from build123d import *
from OCP.BRepFilletAPI import BRepFilletAPI_MakeChamfer

# Parameters (mm, degrees)
BOSS_EXTRUDE1_DEPTH = 40.894
SKETCH3_W           = 13.757082797
SKETCH3_H           = 5.588
CUT_EXTRUDE2_DEPTH  = 40.894
SKETCH6_W           = 7.5565
SKETCH6_H           = 30.48
SKETCH6_H_2         = 7.62
SKETCH6_W_2         = 8.4455
CUT_EXTRUDE4_DEPTH  = 72.423246356
FILLET1_R           = 2.38
FILLET2_R           = 4.92
CHAMFER1_SIZE       = 25.24
CHAMFER1_SIZE2      = 11.769605292
SKETCH9_R           = 3.0988
CUT_EXTRUDE5_DEPTH  = 83.027180008
BOSS_EXTRUDE3_DEPTH = 5.08
BOSS_EXTRUDE4_DEPTH = 5.08
FILLET3_R           = 4.92
FILLET4_R           = 4.92


with BuildPart() as part:
    # Sketch1 → Boss-Extrude1 (new body)
    with BuildSketch(Plane.XY):
        Polygon((66.04, -19.05), (15.24, 19.05), (-15.24, 19.05), (-15.24, 11.43), (10.668, 11.43), (10.668, -19.05), align=None)
    extrude(amount=-BOSS_EXTRUDE1_DEPTH)

    # Sketch3 → Cut-Extrude2 (cut)
    with BuildSketch(Plane(origin=(0, 0, -40.894), x_dir=(-1, 0, 0), z_dir=(0, 0, -1))):
        with Locations((8.361458602, 14.224)):
            Rectangle(SKETCH3_W, SKETCH3_H)
        Polygon((-2.032, 16.256), (-2.032, 19.05), (-13.15212, 19.05), align=None)
    extrude(amount=-CUT_EXTRUDE2_DEPTH, mode=Mode.SUBTRACT)

    # Sketch6 → Cut-Extrude4 (cut, through all)
    with BuildSketch(Plane.ZY.offset(-10.668)):
        with Locations((-35.33775, -3.81)):
            Rectangle(SKETCH6_W, SKETCH6_H)
        with Locations((-35.33775, 15.24)):
            Rectangle(SKETCH6_W, SKETCH6_H_2)
        with Locations((-25.55875, 15.24)):
            Rectangle(SKETCH6_W_2, SKETCH6_H_2)
        with Locations((-25.55875, -3.81)):
            Rectangle(SKETCH6_W_2, SKETCH6_H)
        with Locations((-15.33525, -3.81)):
            Rectangle(SKETCH6_W_2, SKETCH6_H)
        with Locations((-15.33525, 15.24)):
            Rectangle(SKETCH6_W_2, SKETCH6_H_2)
        with Locations((-5.55625, 15.24)):
            Rectangle(SKETCH6_W, SKETCH6_H_2)
        with Locations((-5.55625, -3.81)):
            Rectangle(SKETCH6_W, SKETCH6_H)
    extrude(amount=-CUT_EXTRUDE4_DEPTH, mode=Mode.SUBTRACT)

    # Fillet1
    fillet1_edges = [part.edges().sort_by_distance(p)[0] for p in [
        (66.04, -19.05, -40.005),
        (66.04, -19.05, -30.6705),
        (66.04, -19.05, -20.447),
        (66.04, -19.05, -10.2235),
        (66.04, -19.05, -0.889),
    ]]
    fillet(fillet1_edges, radius=FILLET1_R)

    # Fillet2
    fillet2_edges = [part.edges().sort_by_distance(p)[0] for p in [
        (10.668, -19.05, -40.005),
        (10.668, -19.05, -30.6705),
        (10.668, -19.05, -20.447),
        (10.668, -19.05, -10.2235),
        (10.668, -19.05, -0.889),
    ]]
    fillet(fillet2_edges, radius=FILLET2_R)

    # Chamfer1: one chamfer whose edges measure the first distance from different faces: ONE call of the kernel's chamfer builder (chamfer() names one face for all edges)
    chamfer1_edges_1 = [part.edges().sort_by_distance(p)[0] for p in [
        (10.668, 11.43, -40.005),
    ]]
    chamfer1_side_1 = [part.faces().sort_by_distance(p)[0] for p in [
        (10.668, -1.35, -40.005),
    ]]
    chamfer1_edges_2 = [part.edges().sort_by_distance(p)[0] for p in [
        (10.668, 11.43, -30.6705),
    ]]
    chamfer1_side_2 = [part.faces().sort_by_distance(p)[0] for p in [
        (10.668, -1.35, -30.6705),
    ]]
    chamfer1_edges_3 = [part.edges().sort_by_distance(p)[0] for p in [
        (10.668, 11.43, -20.447),
    ]]
    chamfer1_side_3 = [part.faces().sort_by_distance(p)[0] for p in [
        (10.668, -1.35, -20.447),
    ]]
    chamfer1_edges_4 = [part.edges().sort_by_distance(p)[0] for p in [
        (10.668, 11.43, -10.2235),
    ]]
    chamfer1_side_4 = [part.faces().sort_by_distance(p)[0] for p in [
        (10.668, -1.35, -10.2235),
    ]]
    chamfer1_edges_5 = [part.edges().sort_by_distance(p)[0] for p in [
        (10.668, 11.43, -0.889),
    ]]
    chamfer1_side_5 = [part.faces().sort_by_distance(p)[0] for p in [
        (10.668, -1.35, -0.889),
    ]]
    chamfer1 = BRepFilletAPI_MakeChamfer(part.part.solid().wrapped)
    for e in chamfer1_edges_1:
        chamfer1.Add(CHAMFER1_SIZE, CHAMFER1_SIZE2, e.wrapped, chamfer1_side_1[0].wrapped)  # the first distance lies on this face
    for e in chamfer1_edges_2:
        chamfer1.Add(CHAMFER1_SIZE, CHAMFER1_SIZE2, e.wrapped, chamfer1_side_2[0].wrapped)  # the first distance lies on this face
    for e in chamfer1_edges_3:
        chamfer1.Add(CHAMFER1_SIZE, CHAMFER1_SIZE2, e.wrapped, chamfer1_side_3[0].wrapped)  # the first distance lies on this face
    for e in chamfer1_edges_4:
        chamfer1.Add(CHAMFER1_SIZE, CHAMFER1_SIZE2, e.wrapped, chamfer1_side_4[0].wrapped)  # the first distance lies on this face
    for e in chamfer1_edges_5:
        chamfer1.Add(CHAMFER1_SIZE, CHAMFER1_SIZE2, e.wrapped, chamfer1_side_5[0].wrapped)  # the first distance lies on this face
    add(Compound.cast(chamfer1.Shape()), mode=Mode.REPLACE)

    # Sketch9 → Cut-Extrude5 (cut, through all)
    with BuildSketch(Plane.XZ.offset(-17.018)):
        with Locations(Location((-7.2644, -10.6553, 0), (0, 0, 270))):
            Circle(SKETCH9_R)
        with Locations(Location((-7.2644, -30.2387, 0), (0, 0, 270))):
            Circle(SKETCH9_R)
    extrude(amount=-CUT_EXTRUDE5_DEPTH, mode=Mode.SUBTRACT)

    # Sketch10 → Boss-Extrude3 (add, symmetric)
    with BuildSketch(Plane(origin=(0, 0, -20.447), x_dir=(-1, 0, 0), z_dir=(0, 0, -1))):
        Polygon((1.482917203, 17.018), (15.24, 17.018), (1.482917203, 11.43), align=None)
    extrude(amount=BOSS_EXTRUDE3_DEPTH, both=True)

    # Sketch11 → Boss-Extrude4 (add)
    with BuildSketch(Plane(origin=(0, 0, -40.894), x_dir=(-1, 0, 0), z_dir=(0, 0, -1))):
        Polygon((1.482917203, 17.018), (15.24, 17.018), (1.482917203, 11.43), align=None)
    boss_extrude4 = extrude(amount=-BOSS_EXTRUDE4_DEPTH)

    # Mirror1: Boss-Extrude4 across plane
    add(boss_extrude4.mirror(Plane(origin=(0, 0, -20.447), x_dir=(1, 0, 0), z_dir=(0, 0, -1))))

    # Fillet3
    fillet3_edges = [part.edges().sort_by_distance(p)[0] for p in [
        (10.668, 11.43, -25.55875),
        (10.668, 11.43, -15.33525),
        (10.668, 11.43, -5.55625),
        (10.668, 11.43, -35.33775),
    ]]
    fillet(fillet3_edges, radius=FILLET3_R)

    # Fillet4
    # the kernel refuses this fillet: 4.92 mm, written as the material it adds along each edge
    with BuildSketch(Plane(origin=(-1.101605292, 11.43, 0), x_dir=(-1, 0, 0), z_dir=(0, 0, -1)), Plane(origin=(-1.101605292, 11.43, -39.116), x_dir=(-1, 0, 0), z_dir=(0, 0, -1)), Plane(origin=(-1.101605292, 11.43, -29.7815), x_dir=(-1, 0, 0), z_dir=(0, 0, -1)), Plane(origin=(-1.101605292, 11.43, -19.558), x_dir=(-1, 0, 0), z_dir=(0, 0, -1)), Plane(origin=(-1.101605292, 11.43, -9.3345), x_dir=(-1, 0, 0), z_dir=(0, 0, -1))) as fillet4_piece_1:
        with BuildLine():
            CenterArc((3.761612208, -3.574908377), FILLET4_R, 133.397271211, 21.602728789)
            Line((-0.697422104, -1.495626529), (-0.78660279, -1.454040892))
            Line((-0.78660279, -1.454040892), (-0.089180686, 0.041585637))
            Line((-0.089180686, 0.041585637), (0, 0.0984))
            ThreePointArc((0, 0.0984), (0.190655955, 0.0984), (0.313705905, 0.071498168))
            Line((0.313705905, 0.071498168), (0.381311911, 0))
        make_face()
    extrude(amount=1.778)


solid = part.part
The listing builds one solid part. Answer for the finished solid, in the listing's coordinates (mm). A direction names the side the tool comes from. Give positions to 0.01 mm unless a question says otherwise; leave off trailing zeros. Loops run counter-clockwise (first coordinate to the right, second up) from the corner with the lowest first, then second, coordinate; pieces in that order, holes last. Notation, with made-up numbers: (57, -22.5) - (97, -22.5) arc R17 ccw to (97, 7.5) - close; hole circle Ø8 at (27.5, -32). An arc over 180 degrees is marked (long way). Write each question's results on one line, items separated by ' | '.
1. Consider probe 1 along Z at (x, y) = (21.5, 13); probe 2 along Y at (x, z) = (-11, -26); probe 3 along Y at (x, z) = (0.5, -26). Determine where each line is inside the solid, lowest interval first. Write a range as from..to.
Resolved:
probe 1: z = -40.89..-39.12, -31.56..-29.78, -21.34..-19.56, -11.11..-9.33, -1.78..0 | probe 2: y = 17.02..19.05 | probe 3: y = 11.43..19.05
2. Flat-ended cylindrical pins translate along their axes: P1, Ø8, axis at x = 1, z = -15.5, coming from the -Y side; P2, Ø3.5, axis at x = -7.26, z = -30.24, coming from the +Y side; P3, Ø4, axis at y = 12, z = -16.5, coming from the -X side; P4, Ø1.5, axis at y = -12.5, z = -21, coming from the +X side. Find the tip coordinate at first contact, or state that the pin passes through.
Resolved:
P1: stops at y = 11.43 | P2: passes through | P3: stops at x = -7.81 | P4: stops at x = 58.31
3. Find section B-B, the plane z = -35. Write down the section's boundary in (x, y), then the cut area to 3 significant figures.
Resolved:
outline: (-15.24, 17.02) - (-1.48, 17.02) - (-1.48, 11.43) - (5.75, 11.43) arc R4.92 ccw to (10.67, 16.35) - (10.67, 18.43) - (2.03, 16.26) - (2.03, 19.05) - (-15.24, 19.05) - close | area: 101 mm^2
4. Find section D-D, the plane z = -28. Write down the section's boundary in (x, y).
Resolved:
outline: (-15.24, 17.02) - (-9.41, 17.02) - (-9.41, 19.05) - (-15.24, 19.05) - close; (-5.12, 17.02) - (-1.48, 17.02) - (-1.48, 11.43) - (5.75, 11.43) arc R4.92 ccw to (10.67, 16.35) - (10.67, 18.43) - (2.03, 16.26) - (2.03, 19.05) - (-5.12, 19.05) - close
5. For a pull along Z with two mould halves and no side action, classify faces 5 (the face through (14, 19.05, -20)), 6 (the face through (10.668, 17, -6)), 7 (the face through (10.668, 17, -15)) as +Z half, -Z half, draft (parallel to the pull), parting line (faces both ways), or undercut.
Resolved:
face 5: draft | face 6: undercut | face 7: undercut
6. Find section A-A, the plane x = 56. Write down the section's boundary in (y, z).
Resolved:
outline: (-19.05, -40.89) - (-11.52, -40.89) - (-11.52, -39.12) - (-19.05, -39.12) - close; (-19.05, -31.56) - (-11.52, -31.56) - (-11.52, -29.78) - (-19.05, -29.78) - close; (-19.05, -21.34) - (-11.52, -21.34) - (-11.52, -19.56) - (-19.05, -19.56) - close; (-19.05, -11.11) - (-11.52, -11.11) - (-11.52, -9.33) - (-19.05, -9.33) - close; (-19.05, -1.78) - (-11.52, -1.78) - (-11.52, 0) - (-19.05, 0) - close
7. Find section C-C, the plane y = -9. Write down the section's boundary in (x, z).
Resolved:
outline: (8.43, -40.89) - (52.64, -40.89) - (52.64, -39.12) - (8.43, -39.12) - close; (8.43, -31.56) - (52.64, -31.56) - (52.64, -29.78) - (8.43, -29.78) - close; (8.43, -21.34) - (52.64, -21.34) - (52.64, -19.56) - (8.43, -19.56) - close; (8.43, -11.11) - (52.64, -11.11) - (52.64, -9.33) - (8.43, -9.33) - close; (8.43, -1.78) - (52.64, -1.78) - (52.64, 0) - (8.43, 0) - close
8. Which of the six approach directions +Z, -Z, +X, -X, +Y, -Y give full straight-line access (tool end or side, diameter ignored) to faces 1 (the face through (9.189, 12.833, -15.394)), 2 (the face through (10.668, 17, -26)), 3 (the face through (12.1, -17.6, -0.9)), 4 (the face through (-5, 16, -15.367))?
Resolved:
face 1: +X, -Y | face 2: +X, +Y, -Y | face 3: +Z, -Z, -X, -Y | face 4: -X, -Y
